Geometry: final body of the model. Coordinates: model frame, mm. Face numbers are marked on the shaded views. A direction names the side the tool comes from. Round coordinates to 2 decimals unless told otherwise and drop trailing zeros. Write each loop counter-clockwise with the first axis right and the second up, starting at its lowest first coordinate (ties: lowest second). Pieces come first, ordered by that corner, then holes. Notation, with made-up numbers: M -22.5,-34.5 L 22.5,-34.5 A32 cw 22.5,-1.5 Z; hole C 9,-31 d6. An arc over 180 degrees is marked long. Use one line per item in the form item = value. Start each with the question number.
Item 1: Section query C-C (y = 0.5). Return loops of the section in (x, z), and give its area (3 significant figures).
Item 2: Reachability of the marked faces 4, 5, 6, 7 and 8 from +Z, -Z, +X, -X, +Y, -Y: full face, straight path, thin tool, end or side. Return the list, or none.
Item 3: Section query B-B (x = 32.75). Return loops of the section in (y, z).
Item 4: Section query A-A (z = 32.75). Return loops of the section in (x, y), and give its area (3 significant figures).
Item 5: Section query D-D (z = 12.9). Return loops of the section in (x, y), and give its area (3 significant figures).
Item 6: Ray query, probe 1 along Z at (x, y) = (22.75, 0.7); probe 2 along X at (y, z) = (0.8, 52.6); probe 3 along Y at (x, z) = (11, 53.5). Return the intervals inside material, ascending.
Item 7: Pull-direction query (Z, two-part tool) for the marked faces 1, 2 and 3; classes: pulls with the +Z half, pulls with the -Z half, needs draft (parallel to the pull), parting line crosses it, or undercut.
Item 8: Pin query (flat end, axial travel): pin 1 Ø4 at (y, z) = (-2.5, 48) entering from +X; pin 2 Ø6 at (x, z) = (5, 54.5) entering from +Y; pin 3 Ø3.5 at (x, z) = (-8, 18.5) entering from -Y. Return the tip coordinate at first contact, or that it passes through.
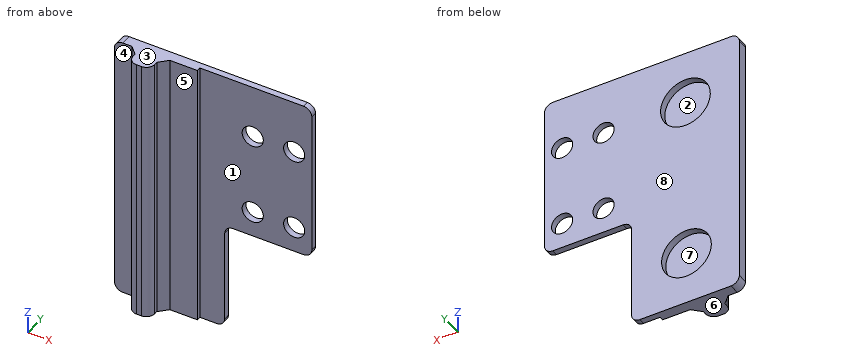
from build123d import *

# Parameters (mm, degrees)
BOSS_EXTRUDE1_DEPTH             = 65.5
CUT_EXTRUDE1_START              = 1.25
SKETCH2_R                       = 6
CUT_EXTRUDE1_DEPTH              = 1.7
BOSS_EXTRUDE2_REACH             = 69.698
SKETCH3_W                       = 21
SKETCH3_H                       = 39
SKETCH3_R                       = 2.55
BOSS_EXTRUDE2_DIRECTION_2_REACH = 69.698
FILLET1_R                       = 2


with BuildPart() as part:
    # Sketch1 → Boss-Extrude1 (new body)
    with BuildSketch(Plane.XY):
        Polygon((-10, -1.25), (-5.8, -1.25), (-3.861348368, -3.188651632), (-3.861348368, -6.058534431), (1.380405129, -6.058534431), (1.380405129, -3.219594871), (3.35, -1.25), (10, -1.25), (10, -0.25), (16, -0.25), (16, 1.25), (10, 1.25), (-10, 1.25), align=None)
    extrude(amount=BOSS_EXTRUDE1_DEPTH)

    # Sketch2 → Cut-Extrude1 (cut)
    with BuildSketch(Plane(origin=(0, 0, 0), x_dir=(1, 0, 0), z_dir=(0, 1, 0)).offset(CUT_EXTRUDE1_START)):
        with Locations(Location((2.75, -12.9, 0), (0, 0, 90))):
            Circle(SKETCH2_R)
        with Locations(Location((3, -52.6, 0), (0, 0, 90))):
            Circle(SKETCH2_R)
    extrude(amount=-CUT_EXTRUDE1_DEPTH, mode=Mode.SUBTRACT)

    # Boss-Extrude2: up to this face of the body (flat: up to its plane)
    boss_extrude2_end = Plane(part.part.faces().sort_by_distance((3.019145607, 1.25, 32.75))[0])
    # Sketch3 → Boss-Extrude2 (add, up to the picked face)
    with BuildSketch(Plane(origin=(0, 0, 0), x_dir=(1, 0, 0), z_dir=(0, 1, 0)), mode=Mode.PRIVATE) as boss_extrude2_sk1:
        with Locations((26.5, -46)):
            Rectangle(SKETCH3_W, SKETCH3_H)
        with Locations(Location((32.75, -52.6, 0), (0, 0, 90))):
            Circle(SKETCH3_R, mode=Mode.SUBTRACT)
        with Locations(Location((32.75, -32.75, 0), (0, 0, 90))):
            Circle(SKETCH3_R, mode=Mode.SUBTRACT)
        with Locations(Location((22.75, -52.6, 0), (0, 0, 90))):
            Circle(SKETCH3_R, mode=Mode.SUBTRACT)
        with Locations(Location((22.75, -32.75, 0), (0, 0, 90))):
            Circle(SKETCH3_R, mode=Mode.SUBTRACT)
    boss_extrude2_tool1 = split(extrude(boss_extrude2_sk1.sketch, amount=BOSS_EXTRUDE2_REACH, mode=Mode.PRIVATE), bisect_by=boss_extrude2_end, keep=Keep.BOTH, mode=Mode.PRIVATE)
    add(boss_extrude2_tool1.solids().sort_by(Axis((26.361464, 0, 46.368507), (0, 1, 0)))[0])

    # Boss-Extrude2 direction 2: up to this face of the body (flat: up to its plane)
    boss_extrude2_direction_2_end = Plane(part.part.faces().sort_by_distance((13, -0.25, 32.75))[0])
    # Sketch3 → Boss-Extrude2 direction 2 (add, up to the picked face)
    with BuildSketch(Plane(origin=(0, 0, 0), x_dir=(1, 0, 0), z_dir=(0, 1, 0)), mode=Mode.PRIVATE) as boss_extrude2_direction_2_sk1:
        with Locations((26.5, -46)):
            Rectangle(SKETCH3_W, SKETCH3_H)
        with Locations(Location((32.75, -52.6, 0), (0, 0, 90))):
            Circle(SKETCH3_R, mode=Mode.SUBTRACT)
        with Locations(Location((32.75, -32.75, 0), (0, 0, 90))):
            Circle(SKETCH3_R, mode=Mode.SUBTRACT)
        with Locations(Location((22.75, -52.6, 0), (0, 0, 90))):
            Circle(SKETCH3_R, mode=Mode.SUBTRACT)
        with Locations(Location((22.75, -32.75, 0), (0, 0, 90))):
            Circle(SKETCH3_R, mode=Mode.SUBTRACT)
    boss_extrude2_direction_2_tool1 = split(extrude(boss_extrude2_direction_2_sk1.sketch, amount=-BOSS_EXTRUDE2_DIRECTION_2_REACH, mode=Mode.PRIVATE), bisect_by=boss_extrude2_direction_2_end, keep=Keep.BOTH, mode=Mode.PRIVATE)
    add(boss_extrude2_direction_2_tool1.solids().sort_by(Axis((26.361464, 0, 46.368507), (0, -1, 0)))[0])

    # Fillet1
    fillet1_edges = [part.edges().sort_by_distance(p)[0] for p in [
        (-10, 0, 65.5),
        (16, 0.5, 0),
        (-10, 0, 0),
        (1.380405129, -6.058534431, 32.75),
        (-3.861348368, -6.058534431, 32.75),
        (37, 0.5, 65.5),
        (37, 0.5, 26.5),
        (16, 0.5, 26.5),
    ]]
    fillet(fillet1_edges, radius=FILLET1_R)


solid = part.part
Working result:
q1.outline = M -10,2 A2 ccw -8,0 L 14,0 A2 ccw 16,2 L 16,24.5 A2 cw 18,26.5 L 35,26.5 A2 ccw 37,28.5 L 37,63.5 A2 ccw 35,65.5 L -8,65.5 A2 ccw -10,63.5 Z; hole C 2.75,12.9 d12; hole C 3,52.6 d12; hole C 22.75,32.75 d5.1; hole C 22.75,52.6 d5.1; hole C 32.75,32.75 d5.1; hole C 32.75,52.6 d5.1
q1.area = 2,210 mm²
q2.face_4 = +Z, -Z, -X, -Y
q2.face_5 = +Z, -Z, +X, -Y
q2.face_6 = -Z, +X, -X, +Y, -Y
q2.face_7 = +Y
q2.face_8 = +Z, -Z, +X, -X, +Y
q3.outline = M -0.25,26.5 L 1.25,26.5 L 1.25,30.2 L -0.25,30.2 Z; M -0.25,35.3 L 1.25,35.3 L 1.25,50.05 L -0.25,50.05 Z; M -0.25,55.15 L 1.25,55.15 L 1.25,65.5 L -0.25,65.5 Z
q4.outline = M -10,-1.25 L -5.8,-1.25 L -3.86,-3.19 L -3.86,-4.06 A2 ccw -1.86,-6.06 L -0.62,-6.06 A2 ccw 1.38,-4.06 L 1.38,-3.22 L 3.35,-1.25 L 10,-1.25 L 10,-0.25 L 20.2,-0.25 L 20.2,1.25 L -10,1.25 Z; M 25.3,-0.25 L 30.2,-0.25 L 30.2,1.25 L 25.3,1.25 Z; M 35.3,-0.25 L 37,-0.25 L 37,1.25 L 35.3,1.25 Z
q4.area = 103 mm²
q5.outline = M -10,-1.25 L -5.8,-1.25 L -3.86,-3.19 L -3.86,-4.06 A2 ccw -1.86,-6.06 L -0.62,-6.06 A2 ccw 1.38,-4.06 L 1.38,-3.22 L 3.35,-1.25 L 10,-1.25 L 10,-0.25 L 16,-0.25 L 16,1.25 L 8.75,1.25 L 8.75,-0.45 L -3.25,-0.45 L -3.25,1.25 L -10,1.25 Z
q5.area = 65.9 mm²
q6.probe_1 = 26.5 to 30.2, 35.3 to 50.05, 55.15 to 65.5
q6.probe_2 = -10 to -3, 9 to 20.2, 25.3 to 30.2, 35.3 to 37
q6.probe_3 = -0.25 to 1.25
q7.face_1 = needs draft
q7.face_2 = undercut
q7.face_3 = pulls with the +Z half
q8.pin_1 = 10
q8.pin_2 = -0.45
q8.pin_3 = -1.25
